The drawing under review shows one solid part. Ordinate dimensions are in mm from its lowest x, y, z. Coordinates: 2 decimals unless noted, no trailing zeros. Order: outer loops, then holes, each group sorted by start corner. A loop starts at its lowest first (then second) coordinate and runs counter-clockwise, first axis right, second up. Notation, with made-up numbers: (70, 84) -> (95, 84) arc R27 cw to (95, 106) -> close; hole circle Ø11 at (22, 72.25). An arc over 180 degrees is marked (long way). Use a Markdown table: item, result. Add a question column.
Q1. Insertion check: pin 1 (1.2 mm diameter, centred on x = 54.63, y = 9.87, fed in from -Z); pin 2 (1 mm diameter, centred on y = 30.5, z = 2.5, fed in from +X); pin 3 (0.9 mm diameter, centred on y = 35, z = 2, fed in from +X); pin 4 (1.5 mm diameter, centred on x = 16, z = 1, fed in from +Y). Each pin has a flat end and moves straight along its axis. Give the tip position at first contact, or say it passes through.
Q2. Add section D-D (z = 0.85). Count the separate pieces of the cut face and the enclosed holes in it, then the cut area to 3 significant figures.
Q3. Add section B-B (x = 46.5). State the section outline as (y, z) points, then the cut area to 3 significant figures.
Q4. Wall thickness on probe 1 along X at (y, z) = (21, 2.05); probe 2 along Y at (x, z) = (46.5, 0.8); probe 3 along X at (y, z) = (19.5, 1.2): over which ranges is each line inside the solid? List them lowest first.
Q5. Add section C-C (x = 26). State the section outline as (y, z) points.
Q6. Add section A-A (y = 18). State the section outline as (x, z) points, then the cut area to 3 significant figures.
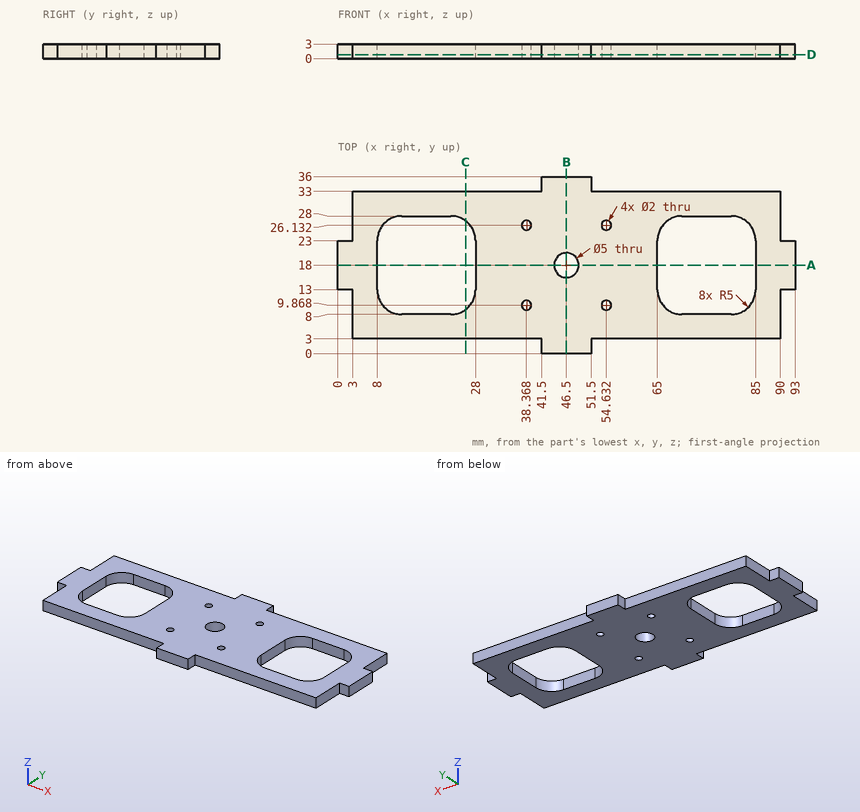
Established:
| question | item | result |
|---|---|---|
| 1 | pin 1 | through |
| 1 | pin 2 | x = 90 |
| 1 | pin 3 | x = 51.5 |
| 1 | pin 4 | y = 33 |
| 2 | separate pieces | 1 |
| 2 | enclosed holes | 7 |
| 2 | area | 1,940 mm^2 |
| 3 | outline | (0, 0) -> (15.5, 0) -> (15.5, 3) -> (0, 3) -> close; (20.5, 0) -> (36, 0) -> (36, 3) -> (20.5, 3) -> close |
| 3 | area | 93.0 mm^2 |
| 4 | probe 1 | 0 to 8, 28 to 65, 85 to 93 |
| 4 | probe 2 | 0 to 15.5, 20.5 to 36 |
| 4 | probe 3 | 0 to 8, 28 to 44.5, 48.5 to 65, 85 to 93 |
| 5 | outline | (3, 0) -> (9, 0) -> (9, 3) -> (3, 3) -> close; (27, 0) -> (33, 0) -> (33, 3) -> (27, 3) -> close |
| 6 | outline | (0, 0) -> (8, 0) -> (8, 3) -> (0, 3) -> close; (28, 0) -> (44, 0) -> (44, 3) -> (28, 3) -> close; (49, 0) -> (65, 0) -> (65, 3) -> (49, 3) -> close; (85, 0) -> (93, 0) -> (93, 3) -> (85, 3) -> close |
| 6 | area | 144 mm^2 |
